Could you check a few things on this drawing? It's one solid part, dimensions in mm from its lowest x, y, z. A direction names the side the tool comes from. Round coordinates to 2 decimals unless told otherwise and drop trailing zeros. Loops run counter-clockwise (first coordinate to the right, second up) from the corner with the lowest first, then second, coordinate; pieces in that order, holes last. Notation, with made-up numbers: (72, 47) -> (129, 47) arc R13 ccw to (129, 63) -> close; hole circle Ø8 at (-36, -36.5). An arc over 180 degrees is marked (long way). Use one line per item in the form item = value. Start each with the question number.
Item 1: If I drill on L1, parallel to Y at x = 38, z = 24.5; L2, parallel to X at y = 20, z = 37.5, over which ranges is the centre line in solid material (lowest first)? Write a range as [from, to].
Item 2: If we section it at C-C (x = 8.5): Write out the boundary of the cut face in (y, z).
Item 3: Thinking about a two-plate mould opening in Z: for the marked faces 4, 5 and 6, which applies, released by +Z, released by -Z, zero draft, split by the parting line, or undercut?
Item 4: If we section it at D-D (y = 18): Write out the boundary of the cut face in (x, z), then the cut area to 3 significant figures.
Item 5: For the marked faces 1, 2 and 3, which set-ups out of +Z, -Z, +X, -X, +Y, -Y let a thin tool reach every point of the face, with its end or its side?
Item 6: If we section it at B-B (y = 67.5): Write out the boundary of the cut face in (x, z), then the cut area to 3 significant figures.
Item 7: If we section it at A-A (z = 23.5): Write out the boundary of the cut face in (x, y), then the cut area to 3 significant figures.
Item 8: I'm going to push flat-ended pins straight in: pin 1 Ø7.5 at (y, z) = (18.5, 31) entering from +X; pin 2 Ø8 at (y, z) = (30, 18) entering from +X; pin 3 Ø3 at (y, z) = (47, 29.5) entering from -X; pin 4 Ø1 at (x, z) = (7.5, 27) entering from +Y. Where does each tip first touch, or does it pass through?
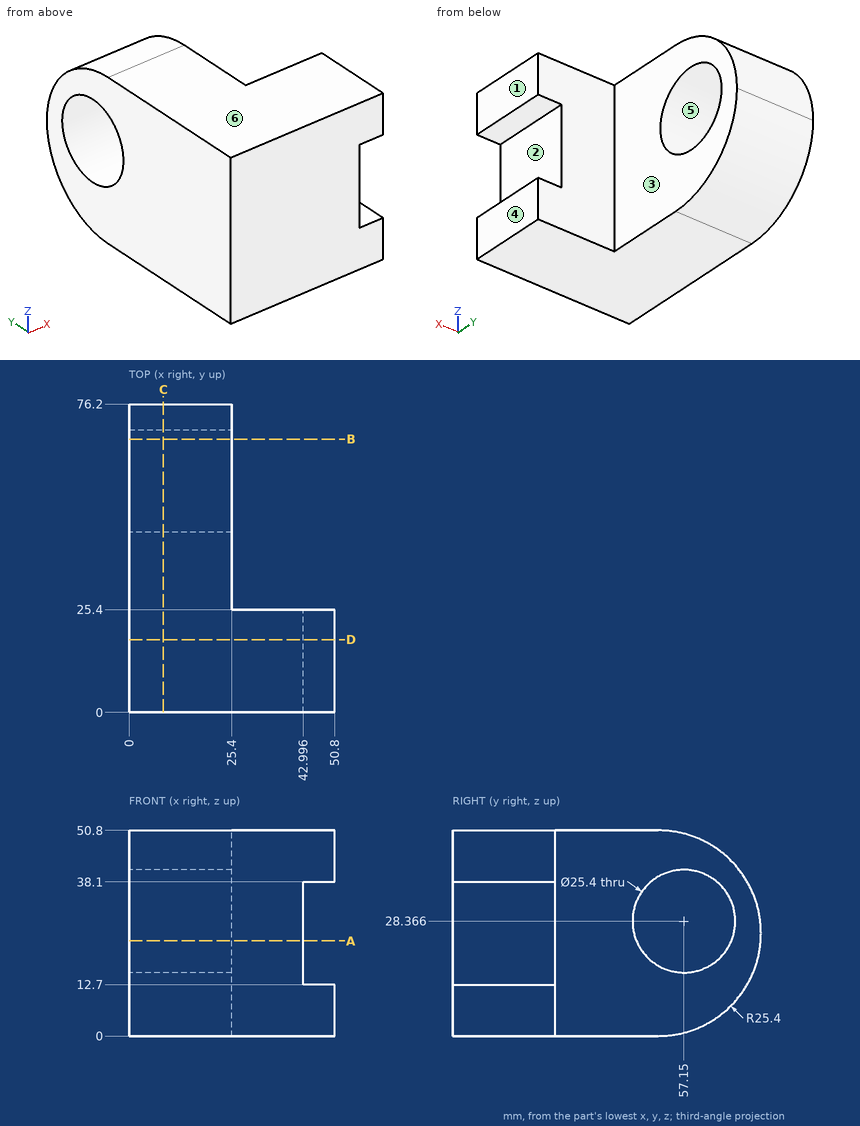
Values found:
q1.L1 = [0, 25.4]
q1.L2 = [0, 43]
q2.outline = (0, 0) -> (50.8, 0) arc R25.4 ccw to (76.2, 25.4) arc R25.4 ccw to (50.8, 50.8) -> (0, 50.8) -> close; hole circle Ø25.4 at (57.15, 28.37)
q3.face_4 = zero draft
q3.face_5 = undercut
q3.face_6 = released by +Z
q4.outline = (0, 0) -> (50.8, 0) -> (50.8, 12.7) -> (43, 12.7) -> (43, 38.1) -> (50.8, 38.1) -> (50.8, 50.8) -> (0, 50.8) -> close
q4.area = 2,380 mm2
q5.face_1 = +Z, -Z, +X, +Y, -Y
q5.face_2 = +X, +Y, -Y
q5.face_3 = +Z, -Z, +X, +Y
q6.outline = (0, 6.26) -> (25.4, 6.26) -> (25.4, 21.01) -> (0, 21.01) -> close; (0, 35.73) -> (25.4, 35.73) -> (25.4, 44.54) -> (0, 44.54) -> close
q6.area = 598 mm2
q7.outline = (0, 0) -> (43, 0) -> (43, 25.4) -> (25.4, 25.4) -> (25.4, 45.42) -> (0, 45.42) -> close; (0, 68.88) -> (25.4, 68.88) -> (25.4, 76.13) -> (0, 76.13) -> close
q7.area = 1,780 mm2
q8.pin_1 = 43
q8.pin_2 = 25.4
q8.pin_3 = through
q8.pin_4 = 76.18
